from build123d import *

# Parameters (mm, degrees)
SKETCH1_W               = 90
SKETCH1_H               = 90.01
BOSS_EXTRUDE1_DEPTH     = 22
SKETCH2_R               = 2
CUT_EXTRUDE1_DEPTH      = 1
CUT_EXTRUDE1_DEPTH_BACK = 23
CUT_EXTRUDE2_DEPTH      = 16.25
SKETCH4_R               = 6.416854585
CUT_EXTRUDE3_DEPTH      = 6.75
CHAMFER1_SIZE           = 1


with BuildPart() as part:
    # Sketch1 → Boss-Extrude1 (new body)
    with BuildSketch(Plane(origin=(0, 0, 0), x_dir=(1, 0, 0), z_dir=(0, 1, 0))):
        with Locations((45, 45.005)):
            Rectangle(SKETCH1_W, SKETCH1_H)
    extrude(amount=BOSS_EXTRUDE1_DEPTH)

    # Sketch2 → Cut-Extrude1 (cut, two sides)
    with BuildSketch(Plane.XZ) as cut_extrude1_sk:
        with Locations((9.997, -7.265579483)):
            Circle(SKETCH2_R)
        with Locations((9.997, -80.01)):
            Circle(SKETCH2_R)
        with Locations((79.997, -7.265579483)):
            Circle(SKETCH2_R)
        with Locations((79.997, -80.01)):
            Circle(SKETCH2_R)
    extrude(amount=CUT_EXTRUDE1_DEPTH, mode=Mode.SUBTRACT)
    extrude(cut_extrude1_sk.sketch, amount=-CUT_EXTRUDE1_DEPTH_BACK, mode=Mode.SUBTRACT)

    # Sketch3 → Cut-Extrude2 (cut)
    with BuildSketch(Plane.XZ):
        with BuildLine():
            Line((26.092808525, -11.764178956), (63.899808525, -11.764178956))
            ThreePointArc((63.899808525, -11.764178956), (82.022370223, -22.681759768), (80.842050765, -43.805861151))
            Line((80.842050765, -43.805861151), (62.765845791, -75.228209836))
            ThreePointArc((62.765845791, -75.228209836), (45.012346751, -85.505995123), (27.242787748, -75.256001397))
            Line((27.242787748, -75.256001397), (8.339287748, -42.514178956))
            ThreePointArc((8.339287748, -42.514178956), (8.339287748, -22.014178956), (26.092808525, -11.764178956))
        make_face()
    extrude(amount=-CUT_EXTRUDE2_DEPTH, mode=Mode.SUBTRACT)

    # Sketch4 → Cut-Extrude3 (cut, through all)
    with BuildSketch(Plane.XZ.offset(-16.25)):
        with Locations((44.996308525, -43.17811977)):
            Circle(SKETCH4_R)
    extrude(amount=-CUT_EXTRUDE3_DEPTH, mode=Mode.SUBTRACT)

    # Chamfer1
    chamfer1_edges = [part.edges().sort_by_distance(p)[0] for p in [
        (7.997, 22, -7.265579483),
        (7.997, 22, -80.01),
        (77.997, 22, -7.265579483),
        (77.997, 22, -80.01),
    ]]
    chamfer(chamfer1_edges, length=CHAMFER1_SIZE)


solid = part.part
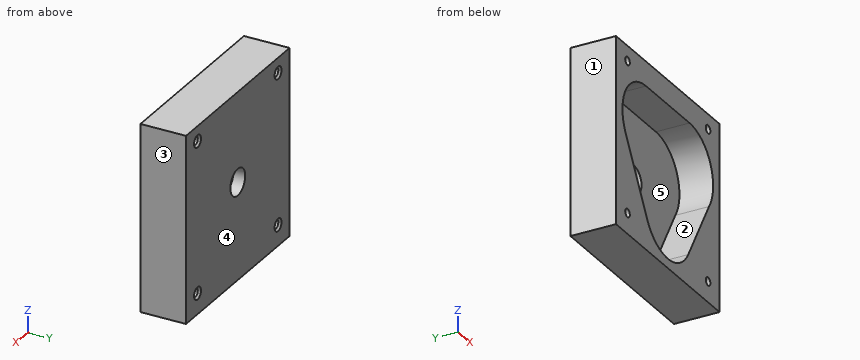
Could you check a few things on this model? Use its own coordinates, in mm. Face numbers are marked on the shaded views. A direction names the side the tool comes from. Coordinates: 2 decimals unless noted, no trailing zeros. Write each loop counter-clockwise with the first axis right and the second up, starting at its lowest first coordinate (ties: lowest second). Pieces come first, ordered by that corner, then holes. Notation, with made-up numbers: (51.5, 13) - (81.5, 13) arc R18 ccw to (81.5, 33) - close; hole circle Ø10 at (-12.75, 80). An arc over 180 degrees is marked (long way). Put each result on its own line as item: value. Start each with the question number.
Q1. Please list where these lines run through material, in increasing order: L1, parallel to Z at x = 45.5, y = 17; L2, parallel to Y at x = 28.5, z = -69; L3, parallel to Z at x = 40.5, y = 17.
Q2. I want a section at B-B on y = 10.5. Write out the boundary of the cut face in (x, z).
Q3. I want a section at D-D on z = -52. Write out the boundary of the cut face in (x, y), plus the area to 3 significant figures.
Q4. I want a section at C-C on x = 22. Write out the boundary of the cut face in (y, z), plus the area to 3 significant figures.
Q5. Which directions (+Z, -Z, +X, -X, +Y, -Y) give clear straight access to the entire face, cutting with the end or side of a thin tool? Please do the marked faces 4 and 5.
Q6. Thinking about a two-plate mould opening in X: for the marked faces 1, 2 and 3, which applies, pulls with the +X half, pulls with the -X half, needs draft (parallel to the pull), parting line crosses it, or undercut?
Q7. I'm going to push flat-ended pins straight in: P1, Ø3, axis at x = 10, z = -7.27, coming from the -Y side; P2, Ø6, axis at x = 28.5, z = -44, coming from the -Y side. Where does each tip first touch, or does it pass through?
Q8. I want a section at A-A on z = -80.01. Write out the boundary of the cut face in (x, y), plus the area to 3 significant figures.
Checks:
1. L1: -90.01 to -49.58, -36.78 to 0
1. L2: 16.25 to 22
1. L3: -90.01 to -47.76, -38.6 to 0
2. outline: (0, -90.01) - (90, -90.01) - (90, 0) - (0, 0) - close; hole circle Ø4 at (10, -80.01); hole circle Ø4 at (10, -7.27); hole (8.34, -42.51) - (27.24, -75.26) arc R20.5 ccw to (62.77, -75.23) - (80.84, -43.81) arc R20.5 ccw to (63.9, -11.76) - (26.09, -11.76) arc R20.5 ccw to start; hole circle Ø4 at (80, -80.01); hole circle Ø4 at (80, -7.27)
3. outline: (0, 0) - (13.82, 0) - (13.82, 16.25) - (76.13, 16.25) - (76.13, 0) - (90, 0) - (90, 22) - (0, 22) - close
3. area: 967 mm²
4. outline: (0, -90.01) - (22, -90.01) - (22, 0) - (0, 0) - (0, -12.18) - (16.25, -12.18) - (16.25, -66.18) - (0, -66.18) - close
4. area: 1,100 mm²
5. face 4: +Z, -Z, +X, -X, +Y
5. face 5: -Y
6. face 1: pulls with the -X half
6. face 2: undercut
6. face 3: pulls with the +X half
7. P1: through
7. P2: y = 16.25
8. outline: (0, 0) - (8, 0) - (8, 21) - (7, 22) - (0, 22) - close; (12, 0) - (31.03, 0) - (31.03, 16.25) - (58.97, 16.25) - (58.97, 0) - (78, 0) - (78, 21) - (77, 22) - (13, 22) - (12, 21) - close; (82, 0) - (90, 0) - (90, 22) - (83, 22) - (82, 21) - close
8. area: 1,350 mm²
